CAD build for the part. Positions are in the model's coordinates, mm. Face numbers are marked on the shaded views. A direction names the side the tool comes from. Give positions to 0.01 mm unless a question says otherwise; leave off trailing zeros. Order: outer loops, then holes, each group sorted by start corner. A loop starts at its lowest first (then second) coordinate and runs counter-clockwise, first axis right, second up. Notation, with made-up numbers: (-21, 2.5) -> (38, 2.5) arc R31 cw to (38, 29.5) -> close; hole circle Ø5 at (-24, 33.25). An arc over 180 degrees is marked (long way). Use one line per item in the form item = value. Start each with the question number.
1) Cut at A-A, the plane z = 14. Give the cut face in (x, y) (3 decimals), and give its area (3 significant figures).
2) Mould opens along Y. For the marked faces 3 and 4 say: pulls with the +Y half, pulls with the -Y half, needs draft (parallel to the pull), parting line crosses it, or undercut.
3) Tool access for the marked faces 1 and 2: list every direction of +Z, -Z, +X, -X, +Y, -Y with a clear straight run to the whole face (end or side of a thin tool).
4) Cut at C-C, the plane y = 10. Give the cut face in (x, z).
5) Cut at D-D, the plane z = -9. Give the cut face in (x, y) (3 decimals), and give its area (3 significant figures).
6) Probe line 1 (Y direction, x = 0, z = -19.75) (3 decimals); line 2 (Z direction, x = -5, y = 2.5); line 3 (X direction, y = 3.5, z = -33.5). List the from-to ranges inside material, lowest first.
7) Drop flat-ended pins along their axis: P1, Ø5, axis at y = -4, z = -20, coming from the -X side; P2, Ø4, axis at x = 4.5, z = 15.5, coming from the +Y side; P3, Ø2, axis at x = 9, z = -2, coming from the -Y side. Give the stop position or say it passes through.
8) Cut at B-B, the plane x = 10.75. Give the cut face in (y, z).
from build123d import *


with BuildPart() as f1:
    # F0 (on Front) → F1 (revolve)
    with BuildSketch(Plane.XZ):
        Polygon((-9.225, 0), (-9.225, 30), (-12.225, 30), (-12.225, -30), (-9.225, -30), align=None)
        Polygon((-9.225, -30), (-4.505, -30), (-4.505, -17.18318), (-9.225, 0), align=None)
        Polygon((-2.275, -17.18318), (-9.225, 0), (-4.505, -17.18318), align=None)
        Polygon((-3.075, 18.308065), (-3.075, 30), (-9.225, 30), (-9.225, 0), (-2.425, 8.714551), align=None)
        Polygon((-12.225, 30), (-9.225, 30), (-9.296466, 37.5), (-12.225, 37.5), align=None)
        Polygon((-9.296466, -37.5), (-9.225, -30), (-12.225, -30), (-12.225, -37.5), align=None)
    revolve(axis=Axis((0, 0, 0), (0, 0, -1)))


solid = f1.part
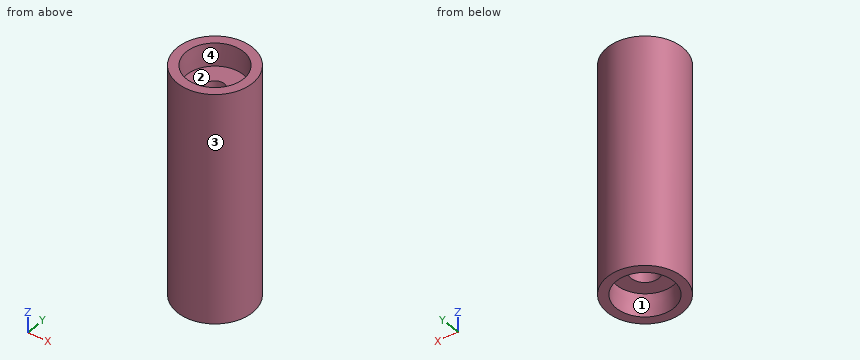
Result:
q1.outline = circle Ø24.45 at (0, 0); hole circle Ø5.566 at (0, 0)
q1.area = 445 mm²
q2.face_3 = parting line crosses it
q2.face_4 = undercut
q3.face_1 = -Z
q3.face_2 = +Z
q4.outline = (-7.03, -37.5) -> (7.03, -37.5) -> (7.03, 37.5) -> (-7.03, 37.5) -> close
q5.outline = circle Ø24.45 at (0, 0); hole circle Ø11.17 at (0, 0)
q5.area = 372 mm²
q6.line_1 = -12.225 to -4.505, 4.505 to 12.225
q6.line_2 = -30 to -8.99, 4.66 to 30
q6.line_3 = -11.71 to -8.57, 8.57 to 11.71
q7.P1 = -12.13
q7.P2 = 11.97
q7.P3 = -9.24
q8.outline = (-5.82, -37.5) -> (5.82, -37.5) -> (5.82, 37.5) -> (-5.82, 37.5) -> close
